CAD build for the part. Positions are in the model's coordinates, mm. Face numbers are marked on the shaded views. A direction names the side the tool comes from. Coordinates: 2 decimals unless noted, no trailing zeros. Loops run counter-clockwise (first coordinate to the right, second up) from the corner with the lowest first, then second, coordinate; pieces in that order, holes last. Notation, with made-up numbers: (44.25, -21.5) -> (48.25, -21.5) arc R25 ccw to (48.25, -5.5) -> close; hole circle Ø3 at (20.5, -14). An arc over 180 degrees is marked (long way). Write each question's results on one line, items separated by ' | '.
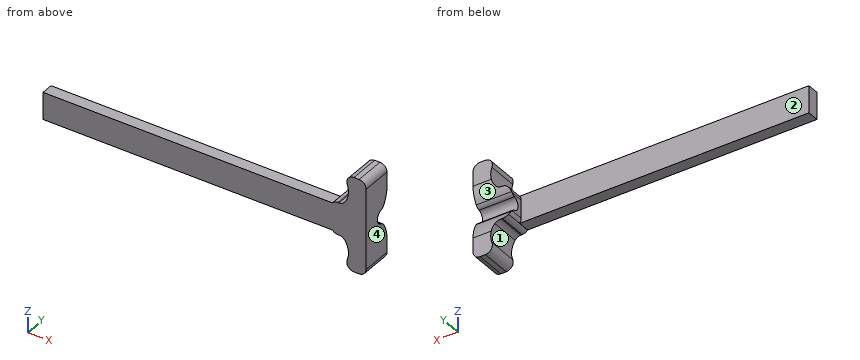
from build123d import *

# Parameters (mm, degrees)
EXTRUDE_1_DEPTH     = 13
EXTRUDE_2_DEPTH     = 5
CUT_EXTRUDE_1_DEPTH = 140.061137634


with BuildPart() as part:
    # Sketch 1 → Extrude 1 (new body)
    with BuildSketch(Plane(origin=(0, 0, 0), x_dir=(1, 0, 0), z_dir=(0, 1, 0))):
        with BuildLine():
            Line((122, 3.83772234), (122, 0))
            Line((122, 0), (137, 0))
            Line((137, 0), (137, 17))
            ThreePointArc((137, 17), (136.121320344, 19.121320344), (134, 20))
            Line((134, 20), (131.781929326, 20))
            ThreePointArc((131.781929326, 20), (129.319163119, 18.713120722), (128.969252111, 15.956521739))
            ThreePointArc((128.969252111, 15.956521739), (129.429754152, 11.909474928), (127.954545455, 8.112843616))
            ThreePointArc((127.954545455, 8.112843616), (126.882997438, 7.175520603), (125.5, 6.83772234))
            Line((125.5, 6.83772234), (125, 6.83772234))
            ThreePointArc((125, 6.83772234), (123.722665467, 6.55220507), (122.68846498, 5.75))
            ThreePointArc((122.68846498, 5.75), (122.177358944, 4.853939575), (122, 3.83772234))
        make_face()
        with BuildLine():
            Line((137, 0), (122, 0))
            Line((122, 0), (122, -3.83772234))
            ThreePointArc((122, -3.83772234), (122.177358944, -4.853939575), (122.68846498, -5.75))
            ThreePointArc((122.68846498, -5.75), (123.722665467, -6.55220507), (125, -6.83772234))
            Line((125, -6.83772234), (125.5, -6.83772234))
            ThreePointArc((125.5, -6.83772234), (126.882997438, -7.175520603), (127.954545455, -8.112843616))
            ThreePointArc((127.954545455, -8.112843616), (129.429754152, -11.909474928), (128.969252111, -15.956521739))
            ThreePointArc((128.969252111, -15.956521739), (129.319163119, -18.713120722), (131.781929326, -20))
            Line((131.781929326, -20), (134, -20))
            ThreePointArc((134, -20), (136.121320344, -19.121320344), (137, -17))
            Line((137, -17), (137, 0))
        make_face()
    extrude(amount=EXTRUDE_1_DEPTH)

    # Sketch 1_3 → Extrude 2 (add)
    with BuildSketch(Plane(origin=(0, 0, 0), x_dir=(1, 0, 0), z_dir=(0, 1, 0))):
        with BuildLine():
            Line((0, 5.75), (0, 0))
            Line((0, 0), (122, 0))
            Line((122, 0), (122, 3.83772234))
            ThreePointArc((122, 3.83772234), (122.177358944, 4.853939575), (122.68846498, 5.75))
            Line((122.68846498, 5.75), (0, 5.75))
        make_face()
        with BuildLine():
            Line((122, 0), (0, 0))
            Line((0, 0), (0, -5.75))
            Line((0, -5.75), (122.68846498, -5.75))
            ThreePointArc((122.68846498, -5.75), (122.177358944, -4.853939575), (122, -3.83772234))
            Line((122, -3.83772234), (122, 0))
        make_face()
    extrude(amount=EXTRUDE_2_DEPTH)

    # Sketch 2 → Cut-Extrude 1 (cut, through all)
    with BuildSketch(Plane(origin=(137, 0, 0), x_dir=(0, 0, -1), z_dir=(1, 0, 0))):
        with BuildLine():
            Line((-10.979609429, 13), (10.979609429, 13))
            ThreePointArc((10.979609429, 13), (7.425251062, 12.484011707), (4.164333864, 10.978645856))
            ThreePointArc((4.164333864, 10.978645856), (3.369802513, 10.222787671), (2.9, 9.231885425))
            ThreePointArc((2.9, 9.231885425), (0, 7), (-2.9, 9.231885425))
            ThreePointArc((-2.9, 9.231885425), (-3.369802513, 10.222787671), (-4.164333864, 10.978645856))
            ThreePointArc((-4.164333864, 10.978645856), (-7.425251062, 12.484011707), (-10.979609429, 13))
        make_face()
    extrude(amount=-CUT_EXTRUDE_1_DEPTH, mode=Mode.SUBTRACT)


solid = part.part
1) Slice it at B-B (x = 38.5). Write the cut outline in (y, z), then the cut area to 3 significant figures.
Outcome:
outline: (0, -5.75) -> (5, -5.75) -> (5, 5.75) -> (0, 5.75) -> close | area: 57.5 mm^2
2) Pin check, flat tips, straight feed: pin 1 (12.5 mm diameter, centred on x = 42.5, z = -1, fed in from +Y); pin 2 (4 mm diameter, centred on x = 74.5, y = 5, fed in from +Z); pin 3 (4.5 mm diameter, centred on y = 7.5, z = -2, fed in from -X). Stop position of each tip, or through.
Outcome:
pin 1: stops at y = 5 | pin 2: stops at z = 5.75 | pin 3: stops at x = 122
3) Which spindle directions (+Z, -Z, +X, -X, +Y, -Y) get a long thin tool onto all of the face, cutting with end or side? Do the marked faces 1 and 2. Say none if no direction does.
Outcome:
face 1: -X, +Y, -Y | face 2: +Z, -Z, -X, +Y
4) Two-plate mould, pull along Z, no slides. Class the marked faces 3 and 4: pulls with the +Z half, pulls with the -Z half, needs draft (parallel to the pull), parting line crosses it, or undercut.
Outcome:
face 3: undercut | face 4: needs draft
5) Drill centre lines: L1, parallel to Z at x = 73, y = 0.75; L2, parallel to Y at x = 109.5, z = 2.5; L3, parallel to X at y = 5, z = 17.5. Where is each one in solid material? Low to high. Write a range as from..to.
Outcome:
L1: z = -5.75..5.75 | L2: y = 0..5 | L3: x = 128.82..136.96
6) Slice it at C-C (y = 1.25). Write the cut outline in (x, z), then the cut area to 3 significant figures.
Outcome:
outline: (0, -5.75) -> (122.69, -5.75) arc R3 ccw to (125, -6.84) -> (125.5, -6.84) arc R3 cw to (127.95, -8.11) arc R8.5 cw to (128.97, -15.96) arc R3 ccw to (131.78, -20) -> (134, -20) arc R3 ccw to (137, -17) -> (137, 17) arc R3 ccw to (134, 20) -> (131.78, 20) arc R3 ccw to (128.97, 15.96) arc R8.5 cw to (127.95, 8.11) arc R3 cw to (125.5, 6.84) -> (125, 6.84) arc R3 ccw to (122.69, 5.75) -> (0, 5.75) -> close | area: 1,810 mm^2
7) Slice it at D-D (z = -9.5). Write the cut outline in (x, y).
Outcome:
outline: (128.75, 0) -> (137, 0) -> (137, 12.91) -> (128.75, 12.91) -> close
8) Slice it at A-A (z = 0). Write the cut outline in (x, y), then the cut area to 3 significant figures.
Outcome:
outline: (0, 0) -> (137, 0) -> (137, 7) -> (122, 7) -> (122, 5) -> (0, 5) -> close | area: 715 mm^2
